Autodesk Inventor part; units mm, degrees
ref_plane "YZ Plane" through (0, 0, 0) normal (1, 0, 0) x (0, 1, 0)
ref_plane "XZ Plane" through (0, 0, 0) normal (0, 1, 0) x (-1, 0, 0)
ref_plane "XY Plane" through (0, 0, 0) normal (0, 0, 1) x (1, 0, 0)
sketch "Sketch1" plane through (0, 0, 0) normal (0, 1, 0) x (-1, 0, 0)
  line L0 (0, 0) -> (0, -16)
  line L1 (8, -8) -> (0, 0)
  line L2 (8, -8) -> (0, -16)
  line L3 (0, 0) -> (-20, 0)
  line L4 (-20, 0) -> (-20, -16)
  line L5 (-20, -16) -> (0, -16)
  dimension "d0" = 16
  dimension "d2" = 20
extrude "Extrusion1" add sketch "Sketch1" along normal blind 5
sketch "Sketch2" plane through (0, 0, 0) normal (0, -1, 0) x (1, 0, 0)
  line L0 (20, -16) -> (0, -16)
  line L1 (20, -16) -> (15, -16)
  line L2 (15, -16) -> (15, 0)
  line L3 (0, 0) -> (20, 0)
  line L4 (20, 0) -> (20, -16)
  line L5 (20, 0) -> (20, -16)
  line L6 (20, -16) -> (18.5, -16)
  line L7 (15, -16) -> (15, -14.5)
  line L8 (15, -16) -> (16.5, -16)
  line L9 (16.5, -14.5) -> (18.5, -14.5)
  line L10 (18.5, -14.5) -> (18.5, -1.5)
  line L11 (18.5, -1.5) -> (16.5, -1.5)
  line L12 (16.5, -1.5) -> (16.5, -14.5)
  dimension "d5" = 5
  dimension "d8" = 1.5
  dimension "d9" = 1.5
  dimension "d11" = 13
extrude "Extrusion2" add sketch "Sketch2" along normal blind 80
extrude "Extrusion3" add sketch "Sketch2" along normal blind 83 contours L12 L11 L10 L9
sketch "Sketch3" plane through (0, 5, 0) normal (0, 1, 0) x (1, 0, 0)
  line L0 (0, 0) -> (20, 0)
  line L1 (20, 16) -> (0, 16)
  line L2 (0, 0) -> (0, 16)
  line L3 (0, 16) -> (-8, 8)
  line L4 (0, 16) -> (-8, 8)
  line L5 (-8, 8) -> (0, 0)
  line L6 (0, 0) -> (-36, 0)
  line L7 (-36, 0) -> (-28, 8)
  line L8 (-28, 8) -> (-36, 16)
  line L9 (-36, 16) -> (0, 16)
  line L10 (-36, 16) -> (-36, 0)
  dimension "d14" = 36
  dimension "d15" = 45
extrude "Extrusion4" add sketch "Sketch3" against normal blind 5 contours L10 L8 L7
sketch "Sketch4" plane through (0, 5, 0) normal (0, 1, 0) x (1, 0, 0)
  line L0 (-28, 8) -> (-36, 0)
  line L1 (20, 16) -> (20, 0)
  line L2 (-36, 0) -> (20, 0)
  line L3 (20, 0) -> (20, 16)
  line L4 (20, 16) -> (-36, 16)
  line L5 (-36, 16) -> (-36, 0)
  line L6 (-36, 8) -> (20, 8)
  line L7 (-28, 8) -> (-8, 8)
  line L8 (-36, 16) -> (-18, 8)
  line L9 (-36, 0) -> (-18, 8)
  line L10 (0, 0) -> (-18, 8)
  line L11 (0, 16) -> (-8, 8)
  line L12 (0, 16) -> (-18, 8)
  line L13 (-27, 12) -> (-9, 12)
  line L14 (-27, 4) -> (-9, 4)
extrude "Extrusion5" add sketch "Sketch4" along normal blind 3 contours L6 L9 L0 | L0 L5 L6 | L6 L5 L8 | L12 L11 L6 | L10 L14 L9 | L6 L1 L2 L10 | L8 L13 L12 | L11 L4 L1 L6
sketch "Sketch5" plane through (0, -80, 0) normal (0, -1, 0) x (1, 0, 0)
  line L0 (15, -16) -> (20, -16)
  line L1 (15, -16) -> (15, 0)
  line L2 (20, -16) -> (15, -16)
  line L3 (15, -16) -> (15, 0)
  line L4 (15, 0) -> (20, 0)
  line L5 (20, 0) -> (20, -16)
  line L6 (18.5, -14.5) -> (16.5, -14.5)
  line L7 (20, -16) -> (18.5, -16)
  line L8 (18.5, -16) -> (18.5, -14.5)
  line L9 (18.5, -14.5) -> (20, -14.5)
  line L10 (20, -14.5) -> (20, -16)
  line L11 (18.5, -1.5) -> (18.5, -14.5)
  line L12 (18.5, -14.5) -> (16.5, -14.5)
  line L13 (16.5, -14.5) -> (16.5, -1.5)
  line L14 (16.5, -1.5) -> (18.5, -1.5)
  line L15 (18.5, -1.5) -> (18.5, -14.5)
  point P0 (0, 0)
properties part number "Connecting pt.1"
Could you check a few things on this model? Use its own coordinates, in mm. A direction names the side the tool comes from. Round coordinates to 2 decimals unless told otherwise and drop trailing zeros. Order: outer loops, then holes, each group sorted by start corner. A loop starts at its lowest first (then second) coordinate and runs counter-clockwise, first axis right, second up. Notation, with made-up numbers: M 74,69 L 117,69 A24 cw 117,84 Z; hole C -30.75,31.5 d7. An arc over 180 degrees is marked long. One line per item, written item: value.
(1) I need wall thicknesses on line 1 along Y through (x, z) = (15.5, -4.25); line 2 along X through (y, z) = (-77.5, -3.75); line 3 along Y through (x, z) = (2.5, -13). Which ranges of each line are inside material? Lowest first, please. Write a range as from..to.
Ans:
line 1: y = -80..8
line 2: x = 15..20
line 3: y = 0..8
(2) Imagine slicing it at B-B (y = -31). Write out the boundary of the cut face in (x, z).
Ans:
outline: M 15,-16 L 20,-16 L 20,0 L 15,0 Z
(3) I'm going to push flat-ended pins straight in: P1, Ø1.6, axis at x = 17, y = -82, coming from the -Z side; P2, Ø1, axis at x = 17.5, y = -81.5, coming from the +Z side; P3, Ø5, axis at x = -26.5, z = -5, coming from the -Y side. Where does each tip first touch, or does it pass through?
Ans:
P1: stops at z = -14.5
P2: stops at z = -1.5
P3: stops at y = 5
(4) Imagine slicing it at C-C (x = -16.5). Write out the boundary of the cut face in (y, z), and give its area (3 significant figures).
Ans:
outline: M 5,-12 L 8,-12 L 8,-4 L 5,-4 Z
area: 24.0 mm^2
(5) Imagine slicing it at A-A (z = -9.75). Write out the boundary of the cut face in (x, y), and give its area (4 significant figures).
Ans:
outline: M -36,0 L -29.75,0 L -29.75,5 L -6.25,5 L -6.25,0 L 15,0 L 15,-80 L 16.5,-80 L 16.5,-83 L 18.5,-83 L 18.5,-80 L 20,-80 L 20,8 L -36,8 Z
area: 736.5 mm^2
(6) Which directions (+Z, -Z, +X, -X, +Y, -Y) give clear straight access to the entire face, cutting with the end or side of a thin tool? Please do faces 1 (the flat face through (-31.563, 6.479, -14.028)), 2 (the flat face through (18, -81, -1.5)), 3 (the flat face through (16.5, -81, -8)), 4 (the flat face through (-31.563, 6.479, -1.972)).
Ans:
face 1: -Z, +Y, -Y
face 2: +Z, +X, -X, -Y
face 3: +Z, -Z, -X, -Y
face 4: +Z, +Y, -Y
